Autodesk Inventor part; units mm, degrees
ref_plane "YZ Plane" through (0, 0, 0) normal (1, 0, 0) x (0, 1, 0)
ref_plane "XZ Plane" through (0, 0, 0) normal (0, 1, 0) x (-1, 0, 0)
ref_plane "XY Plane" through (0, 0, 0) normal (0, 0, 1) x (1, 0, 0)
sketch "Sketch1" plane through (0, 0, 0) normal (0, 1, 0) x (-1, 0, 0)
  line L0 (98.75, 112.5) -> (-98.75, 112.5)
  line L1 (-98.75, 112.5) -> (-98.75, -112.5)
  line L2 (-98.75, -112.5) -> (98.75, -112.5)
  line L3 (98.75, -112.5) -> (98.75, 112.5)
  line L4 (98.75, 112.5) -> (-98.75, -112.5) construction
  line L5 (-98.75, 112.5) -> (98.75, -112.5) construction
  point P0 (0, 0)
  dimension "d0" = 197.5
  dimension "d1" = 225
extrude "Extrusion1" add sketch "Sketch1" along normal blind 100
shell "Shell1" thickness 5 removed faces 1 at (32.9167, 100, 37.5)
sketch "Sketch2" plane through (-93.75, 5, -107.5) normal (0, 1, 0) x (1, 0, 0)
  circle A0 centre (10, -15) radius 1.5
  line L0 (187.5, -215) -> (0, -215)
  line L1 (93.75, -215) -> (93.75, 0)
  line L2 (0, 0) -> (187.5, 0)
  line L3 (187.5, -215) -> (187.5, 0)
  line L4 (0, -215) -> (0, 0)
  line L5 (192.5, 5) -> (-5, 5)
  circle A1 centre (10, -205.267) radius 1.5
  circle A2 centre (177.5, -15) radius 1.5
  circle A3 centre (177.5, -205.267) radius 1.5
  point P0 (93.75, -107.5)
  dimension "d5" = 3
  dimension "d6" = 20
  dimension "d7" = 3
  dimension "d8" = 190.267
  dimension "d9" = 10
extrude "Extrusion2" cut sketch "Sketch2" against normal through all contours A0 | A1 | A2 | A3
properties part number "Box"
Source: CAD feature listing. Evaluate the final solid. Frame: model axes, mm. A direction names the side the tool comes from. Give positions to 0.01 mm unless a question says otherwise; leave off trailing zeros. Order: outer loops, then holes, each group sorted by start corner. A loop starts at its lowest first (then second) coordinate and runs counter-clockwise, first axis right, second up. Notation, with made-up numbers: (59.25, -34.5) -> (112.25, -34.5) arc R10 ccw to (112.25, -16.5) -> close; hole circle Ø1 at (5.25, 39.25). An arc over 180 degrees is marked (long way). Write item = value, one per line.
Item 1: Ray query, probe 1 along Z at (x, y) = (-83.75, 1.15); probe 2 along Z at (x, y) = (29, 35); probe 3 along X at (y, z) = (2.4, -92.5). Return the intervals inside material, ascending.
Check result:
probe_1 = -112.5 to -94, -91 to 96.27, 99.27 to 112.5
probe_2 = -112.5 to -107.5, 107.5 to 112.5
probe_3 = -98.75 to -85.25, -82.25 to 82.25, 85.25 to 98.75
Item 2: Section query A-A (y = 46). Output: boundary loops of the cut face in (x, z).
Check result:
outline = (-98.75, -112.5) -> (98.75, -112.5) -> (98.75, 112.5) -> (-98.75, 112.5) -> close; hole (-93.75, -107.5) -> (93.75, -107.5) -> (93.75, 107.5) -> (-93.75, 107.5) -> close
Item 3: Section query B-B (x = 36). Output: boundary loops of the cut face in (y, z), then the cut area to 4 significant figures.
Check result:
outline = (0, -112.5) -> (100, -112.5) -> (100, -107.5) -> (5, -107.5) -> (5, 107.5) -> (100, 107.5) -> (100, 112.5) -> (0, 112.5) -> close
area = 2,075 mm²
Item 4: Section query C-C (z = 34.5). Output: boundary loops of the cut face in (x, y).
Check result:
outline = (-98.75, 0) -> (98.75, 0) -> (98.75, 100) -> (93.75, 100) -> (93.75, 5) -> (-93.75, 5) -> (-93.75, 100) -> (-98.75, 100) -> close
Item 5: Set-up query: faces 1 (the face through (-1, 49, 112.5)), 2 (the face through (1, 5, 2)). Return all of +Z, -Z, +X, -X, +Y, -Y with unobstructed straight access to the full face (end or side cutting, diameter ignored); none if empty.
Check result:
face_1 = +Z, +X, -X, +Y, -Y
face_2 = +Y
Item 6: Contact query for a flat-ended pin moving along its axis: pin 1 (4 mm diameter, centred on x = -83.75, z = 97.767, fed in from +Y). Output: stop coordinate, or through.
Check result:
pin_1 = 5
Item 7: Mould query, pull axis X, two halves, no side actions, for faces 3 (the face through (-93.75, 52, -2)), 4 (the face through (-98.75, 49, -2)), 5 (the face through (1, 0, 2)). Classes: +X half, -X half, draft (parallel to the pull), parting line (faces both ways), or undercut.
Check result:
face_3 = undercut
face_4 = -X half
face_5 = draft
